from build123d import *

# Parameters (mm, degrees)
SALIENTE_EXTRUIR1_DEPTH = 5
REDONDEO1_R             = 5
CROQUIS3_R              = 1.55
CROQUIS3_R_2            = 2.55
CORTAR_EXTRUIR1_DEPTH   = 269.118443976
REDONDEO3_R             = 25


with BuildPart() as part:
    # Croquis2 → Saliente-Extruir1 (new body)
    with BuildSketch(Plane(origin=(0, 0, 0), x_dir=(1, 0, 0), z_dir=(0, 1, 0))):
        Polygon((-267.5, 8), (-235.5, 8), (-235.5, -8), (-267.5, -8), (-267.5, -17.5), (-225.5, -17.5), (-199.75, -8.5), (-59.75, -8.5), (-34, -17.5), (34, -17.5), (59.75, -8.5), (199.75, -8.5), (225.5, -17.5), (267.5, -17.5), (267.5, -8), (235.5, -8), (235.5, 8), (267.5, 8), (267.5, 17.5), (225.5, 17.5), (199.75, 8.5), (59.75, 8.5), (34, 17.5), (-34, 17.5), (-59.75, 8.5), (-199.75, 8.5), (-225.5, 17.5), (-267.5, 17.5), align=None)
        with BuildLine():
            Line((-204.02626503, 4.698013204), (-223.850289247, 11.626798368))
            ThreePointArc((-223.850289247, 11.626798368), (-228.394084159, 10.984080534), (-230.5, 6.906792602))
            Line((-230.5, 6.906792602), (-230.5, -6.906792602))
            ThreePointArc((-230.5, -6.906792602), (-228.394084159, -10.984080534), (-223.850289247, -11.626798368))
            Line((-223.850289247, -11.626798368), (-204.02626503, -4.698013204))
            ThreePointArc((-204.02626503, -4.698013204), (-200.737601329, 0), (-204.02626503, 4.698013204))
        make_face(mode=Mode.SUBTRACT)
        with BuildLine():
            Line((204.02626503, 4.698013204), (223.850289247, 11.626798368))
            ThreePointArc((223.850289247, 11.626798368), (228.394084159, 10.984080534), (230.5, 6.906792602))
            Line((230.5, 6.906792602), (230.5, -6.906792602))
            ThreePointArc((230.5, -6.906792602), (228.394084159, -10.984080534), (223.850289247, -11.626798368))
            Line((223.850289247, -11.626798368), (204.02626503, -4.698013204))
            ThreePointArc((204.02626503, -4.698013204), (200.737601329, 0), (204.02626503, 4.698013204))
        make_face(mode=Mode.SUBTRACT)
    extrude(amount=SALIENTE_EXTRUIR1_DEPTH)

    # Redondeo1
    redondeo1_edges = [part.edges().sort_by_distance(p)[0] for p in [
        (235.5, 2.5, -8),
        (235.5, 2.5, 8),
        (267.5, 2.5, 17.5),
        (-267.5, 2.5, 17.5),
        (-235.5, 2.5, 8),
        (-235.5, 2.5, -8),
        (-267.5, 2.5, -17.5),
        (267.5, 2.5, -17.5),
    ]]
    fillet(redondeo1_edges, radius=REDONDEO1_R)

    # Croquis3 → Cortar-Extruir1 (cut, through all)
    with BuildSketch(Plane(origin=(0, 5, 0), x_dir=(1, 0, 0), z_dir=(0, 1, 0))):
        with Locations(Location((-264, -12.5, 0), (0, 0, 270))):
            Circle(CROQUIS3_R)
        with Locations(Location((-239, -12.5, 0), (0, 0, 270))):
            Circle(CROQUIS3_R)
        with Locations(Location((-239, 12.5, 0), (0, 0, 270))):
            Circle(CROQUIS3_R)
        with Locations(Location((-264, 12.5, 0), (0, 0, 270))):
            Circle(CROQUIS3_R)
        with Locations(Location((264, 12.5, 0), (0, 0, 90))):
            Circle(CROQUIS3_R)
        with Locations(Location((239, 12.5, 0), (0, 0, 90))):
            Circle(CROQUIS3_R)
        with Locations(Location((239, -12.5, 0), (0, 0, 90))):
            Circle(CROQUIS3_R)
        with Locations(Location((264, -12.5, 0), (0, 0, 90))):
            Circle(CROQUIS3_R)
        with Locations(Location((-18, -11, 0), (0, 0, 270))):
            Circle(CROQUIS3_R_2)
        with Locations(Location((20, -11, 0), (0, 0, 270))):
            Circle(CROQUIS3_R_2)
        with Locations(Location((20, 11, 0), (0, 0, 270))):
            Circle(CROQUIS3_R_2)
        with Locations(Location((-18, 11, 0), (0, 0, 270))):
            Circle(CROQUIS3_R_2)
    extrude(amount=-CORTAR_EXTRUIR1_DEPTH, mode=Mode.SUBTRACT)

    # Redondeo3
    redondeo3_edges = [part.edges().sort_by_distance(p)[0] for p in [
        (225.5, 2.5, 17.5),
        (199.75, 2.5, 8.5),
        (59.75, 2.5, 8.5),
        (34, 2.5, 17.5),
        (-34, 2.5, 17.5),
        (-59.75, 2.5, 8.5),
        (-199.75, 2.5, 8.5),
        (-225.5, 2.5, 17.5),
        (-225.5, 2.5, -17.5),
        (-199.75, 2.5, -8.5),
        (-59.75, 2.5, -8.5),
        (-34, 2.5, -17.5),
        (34, 2.5, -17.5),
        (59.75, 2.5, -8.5),
        (199.75, 2.5, -8.5),
        (225.5, 2.5, -17.5),
    ]]
    fillet(redondeo3_edges, radius=REDONDEO3_R)


solid = part.part
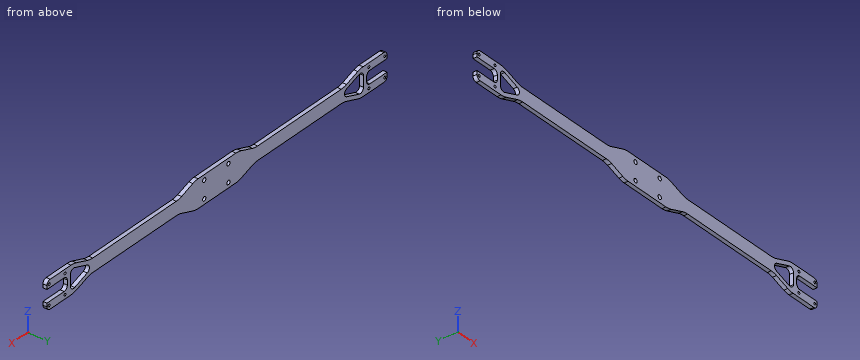
CAD build for the part. Positions are in the model's coordinates, mm. Coordinates: 2 decimals unless noted, no trailing zeros. Order: outer loops, then holes, each group sorted by start corner. A loop starts at its lowest first (then second) coordinate and runs counter-clockwise, first axis right, second up.
Item 1: Drill centre lines: L1, parallel to X at y = 1.4, z = -0.5; L2, parallel to Z at x = -101, y = 2.65; L3, parallel to Z at x = 51.5, y = 4. Where is each one in solid material? Low to high.
Check sheet entries:
L1: x = -235.5 to -230.5, -200.76 to 200.76, 230.5 to 235.5
L2: z = -8.5 to 8.5
L3: z = -11.38 to 11.38
Item 2: Band-saw the part on A-A on y = 3.25. Give the number of separate pieces and of enclosed holes in the cut face, plus the area to 3 significant figures.
Check sheet entries:
separate pieces: 1
enclosed holes: 14
area: 10,600 mm2
Item 3: Pin check, flat tips, straight feed: pin 1 Ø2 at (x, y) = (-204.5, 0.5) entering from -Z; pin 2 Ø1.5 at (y, z) = (2, 4.5) entering from +X; pin 3 Ø2.5 at (y, z) = (2.5, 1.5) entering from -X. Stop position of each tip, or through.
Check sheet entries:
pin 1: stops at z = -10.51
pin 2: stops at x = 236.03
pin 3: stops at x = -235.5
Item 4: Band-saw the part on B-B on x = 156. List the corners of the cut face in (y, z).
Check sheet entries:
outline: (0, -8.5) - (5, -8.5) - (5, 8.5) - (0, 8.5) - close
